from build123d import *

# Parameters (mm, degrees)
SKETCH_1_R                = 20
SKETCH_1_R_2              = 11.1
EXTRUDE_1_DEPTH           = 60
EXTRUDE_2_DEPTH           = 30
SKETCH_4_R                = 11
EXTRUDE_3_DEPTH           = 5
SKETCH_8_R                = 11.1
CUT_EXTRUDE_1_DEPTH       = 100
FILLET_4_R                = 20
EXTRUDE_START             = -30
SKETCH_18_R               = 35
EXTRUDE_4_DEPTH           = 5
EXTRUDE_START_2           = -25
SKETCH_19_R               = 35
EXTRUDE_5_DEPTH           = 5
FILLET_5_R                = 10
CUT_EXTRUDE_9_DEPTH       = 388.169213652
CUT_EXTRUDE_9_DEPTH_BACK  = 388.169213652
SKETCH_21_R               = 2.6
CUT_EXTRUDE_10_DEPTH      = 409.372938359
CUT_EXTRUDE_10_DEPTH_BACK = 409.372938359
SKETCH_22_W               = 35
SKETCH_22_H               = 453.381241258
SKETCH_22_W_2             = 30
SKETCH_22_H_2             = 431.087956996


with BuildPart() as part:
    # 草图1 → 凸台-拉伸1 (new body)
    with BuildSketch(Plane.XY):
        Circle(SKETCH_1_R)
        Circle(SKETCH_1_R_2, mode=Mode.SUBTRACT)
    extrude(amount=EXTRUDE_1_DEPTH)

    # 草图2 → 凸台-拉伸2 (add, symmetric)
    with BuildSketch(Plane.XY.offset(30)):
        with BuildLine():
            Line((-14.142135624, 14.142135624), (-90, -61.715728753))
            Line((-90, -61.715728753), (-90, -320))
            Line((-90, -320), (-50, -320))
            Line((-50, -320), (-50, -78.284271247))
            Line((-50, -78.284271247), (14.142135624, -14.142135624))
            ThreePointArc((14.142135624, -14.142135624), (-14.142135624, -14.142135624), (-14.142135624, 14.142135624))
        make_face()
    extrude(amount=EXTRUDE_2_DEPTH, both=True)

    # 草图4 → 凸台-拉伸3 (add)
    with BuildSketch(Plane.XY.offset(60)):
        with BuildLine():
            Line((-90, -290), (-50, -290))
            Line((-50, -290), (-50, -350))
            ThreePointArc((-50, -350), (-70, -370), (-90, -350))
            Line((-90, -350), (-90, -290))
        make_face()
        with Locations((-70, -350)):
            Circle(SKETCH_4_R, mode=Mode.SUBTRACT)
    extrude_3 = extrude(amount=EXTRUDE_3_DEPTH)

    # 镜向1: 凸台-拉伸3 across plane
    add(extrude_3.mirror(Plane.XY.offset(30)))

    # 草图8 → 切除-拉伸1 (cut)
    with BuildSketch(Plane.XY.offset(60)):
        with Locations((-35.355339059, -35.355339059)):
            Circle(SKETCH_8_R)
    extrude(amount=-CUT_EXTRUDE_1_DEPTH, mode=Mode.SUBTRACT)

    # 圆角4
    fillet_4_edges = [part.edges().sort_by_distance(p)[0] for p in [
        (-50, -78.284271247, 30),
        (-90, -61.715728753, 30),
    ]]
    fillet(fillet_4_edges, radius=FILLET_4_R)

    # 草图18 → 凸台-拉伸4 (add)
    with BuildSketch(Plane.XY.offset(60).offset(EXTRUDE_START)):
        with BuildLine():
            ThreePointArc((16.783988507, -10.876475983), (15.54903282, -12.578854413), (14.142135624, -14.142135624))
            Line((14.142135624, -14.142135624), (-44.142135624, -72.426406871))
            ThreePointArc((-44.142135624, -72.426406871), (-48.47759065, -78.914873848), (-50, -86.568542495))
            Line((-50, -86.568542495), (-50, -129.282056212))
            Line((-50, -129.282056212), (24.135744866, -129.282056212))
            ThreePointArc((24.135744866, -129.282056212), (66.634203362, -100.885494101), (56.662656801, -50.755144277))
            Line((56.662656801, -50.755144277), (16.783988507, -10.876475983))
        make_face()
        with Locations((24.135744866, -83.282056212)):
            Circle(SKETCH_18_R, mode=Mode.SUBTRACT)
    extrude(amount=EXTRUDE_4_DEPTH)

    # 草图19 → 凸台-拉伸5 (add)
    with BuildSketch(Plane(origin=(0, 0, 0), x_dir=(-1, 0, 0), z_dir=(0, 0, -1)).offset(EXTRUDE_START_2)):
        with BuildLine():
            Line((50, -135.340123781), (50, -227.340123781))
            Line((50, -227.340123781), (-4.524131353, -227.340123781))
            ThreePointArc((-4.524131353, -227.340123781), (-50.524131353, -181.340123781), (-4.524131353, -135.340123781))
            Line((-4.524131353, -135.340123781), (50, -135.340123781))
        make_face()
        with Locations((-4.524131353, -181.340123781)):
            Circle(SKETCH_19_R, mode=Mode.SUBTRACT)
    extrude(amount=-EXTRUDE_5_DEPTH)

    # 圆角5
    # the kernel refuses this fillet: 10 mm, written as the material it adds along each edge
    with BuildSketch(Plane(origin=(-50, -227.340123781, 25), x_dir=(0, -1, 0), z_dir=(0, 0, 1)), Plane(origin=(-50, -129.282056212, 30), x_dir=(0, -1, 0), z_dir=(0, 0, 1))) as fillet_5_piece_1:
        with BuildLine():
            CenterArc((FILLET_5_R, FILLET_5_R), FILLET_5_R, 180, 90)
            Line((0, FILLET_5_R), (0, 0))
            Line((0, 0), (FILLET_5_R, 0))
        make_face()
    extrude(amount=5)

    # 草图21 → 切除-拉伸9 (cut, two sides: drawn at the far end of the back side and taken through both)
    with BuildSketch(Plane.XY.offset(65).offset(-CUT_EXTRUDE_9_DEPTH_BACK)):
        with Locations((-70, -75)):
            Circle(SKETCH_21_R)
        with Locations((-70, -250)):
            Circle(SKETCH_21_R)
        with Locations((-58, -300)):
            Circle(SKETCH_21_R)
        with Locations((-82, -300)):
            Circle(SKETCH_21_R)
    extrude(amount=CUT_EXTRUDE_9_DEPTH + CUT_EXTRUDE_9_DEPTH_BACK, mode=Mode.SUBTRACT)

    # 草图22 → 切除-拉伸10 (cut, two sides: drawn at the far end of the back side and taken through both)
    with BuildSketch(Plane.ZY.offset(90).offset(-CUT_EXTRUDE_10_DEPTH_BACK)):
        with Locations((12.5, -161.772701044)):
            Rectangle(SKETCH_22_W, SKETCH_22_H)
        with Locations((50, -154.456021502)):
            Rectangle(SKETCH_22_W_2, SKETCH_22_H_2)
    extrude(amount=CUT_EXTRUDE_10_DEPTH + CUT_EXTRUDE_10_DEPTH_BACK, mode=Mode.SUBTRACT)


solid = part.part
The listing builds one solid part. Answer for the finished solid, in the listing's coordinates (mm). Give positions to 0.01 mm unless a question says otherwise; leave off trailing zeros. Loops run counter-clockwise (first coordinate to the right, second up) from the corner with the lowest first, then second, coordinate; pieces in that order, holes last.
Item 1: Find the intervals of material crossed by line 1 along X through (y, z) = (-300, 33.45); line 2 along Y through (x, z) = (-70, 31.85); line 3 along Y through (x, z) = (0, 30.3), in increasing order.
Derived:
line 1: x = -90 to -84.6, -79.4 to -60.6, -55.4 to -50
line 2: y = -320 to -252.6, -247.4 to -77.6, -72.4 to -41.72
line 3: y = -129.28 to -108.63, -57.94 to -11.1, 11.1 to 20
Item 2: A cutting plane is placed at C-C (z = 33.9). Give the vertices of the cut face in (x, y).
Derived:
outline: (-90, -320) - (-50, -320) - (-50, -139.28) arc R10 cw to (-40, -129.28) - (24.14, -129.28) arc R46 ccw to (56.66, -50.76) - (16.78, -10.88) arc R20 ccw to (-14.14, 14.14) - (-84.14, -55.86) arc R20 ccw to (-90, -70) - close; hole circle Ø5.2 at (-82, -300); hole circle Ø5.2 at (-70, -250); hole circle Ø5.2 at (-70, -75); hole circle Ø5.2 at (-58, -300); hole circle Ø22.2 at (-35.36, -35.36); hole circle Ø22.2 at (0, 0); hole circle Ø70 at (24.14, -83.28)
Item 3: A cutting plane is placed at B-B (y = 0). Give the vertices of the cut face in (x, z), then the cut area to 3 significant figures.
Derived:
outline: (-28.28, 30) - (-11.1, 30) - (-11.1, 35) - (-28.28, 35) - close; (11.1, 30) - (20, 30) - (20, 35) - (11.1, 35) - close
area: 130 mm2
Item 4: Determine the mould class of faces 1 (the cylindrical face through (40.29, -114.33, 32.47)), 2 (the cylindrical face through (12.895, 15.288, 32.465)), 3 (the cylindrical face through (66.34, -101.58, 32.47)), 4 (the flat face through (-48.652, -20.368, 32.535)) for opening direction X: +X half, -X half, draft (parallel to the pull), parting line (faces both ways), or undercut.
Derived:
face 1: undercut
face 2: parting line
face 3: +X half
face 4: -X half
Item 5: A cutting plane is placed at D-D (x = 0). Give the vertices of the cut face in (y, z).
Derived:
outline: (-129.28, 30) - (-108.63, 30) - (-108.63, 35) - (-129.28, 35) - close; (-57.94, 30) - (-11.1, 30) - (-11.1, 35) - (-57.94, 35) - close; (11.1, 30) - (20, 30) - (20, 35) - (11.1, 35) - close
Item 6: A cutting plane is placed at A-A (x = 32.5). Give the vertices of the cut face in (y, z).
Derived:
outline: (-128.52, 30) - (-117.27, 30) - (-117.27, 35) - (-128.52, 35) - close; (-49.3, 30) - (-26.59, 30) - (-26.59, 35) - (-49.3, 35) - close
Item 7: This flat-tipped pin is pushed along its axis until it touches: pin 1 Ø2.5 at (y, z) = (-242, 31.5) entering from +X. Where does it stop, or does it pass through?
Derived:
pin 1: stops at x = -50
